Geometry: final body of the model. Coordinates: model frame, mm. Face numbers are marked on the shaded views. Give positions to 0.01 mm unless a question says otherwise; leave off trailing zeros. Loops run counter-clockwise (first coordinate to the right, second up) from the corner with the lowest first, then second, coordinate; pieces in that order, holes last. Notation, with made-up numbers: M -8.5,40.5 L 5.5,40.5 A13 cw 5.5,44.5 Z; hole C -38.75,71 d4. An arc over 180 degrees is marked long. Put each result on its own line as item: value.
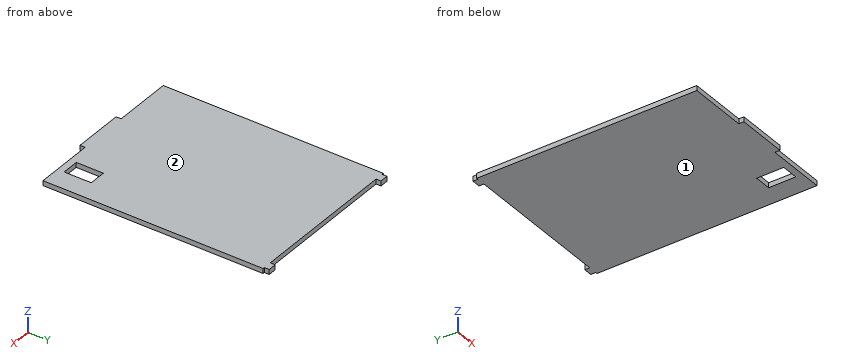
```python
from build123d import *

# Parameters (mm, degrees)
EXTRUDE_1_DEPTH = 2.9


with BuildPart() as part:
    # 草图1 → 凸台-拉伸1 (new body)
    with BuildSketch(Plane.XY):
        Polygon((65, -3), (65, 0), (100, 0), (100, 130), (99, 130), (99, 132.9), (95, 132.9), (94, 132.9), (94, 130), (6, 130), (6, 132.9), (5, 132.9), (1, 132.9), (1, 130), (0, 130), (0, 0), (35, 0), (35, -3), (50, -3), align=None)
        Polygon((83, 4), (78, 4), (78, 20), (83, 20), (88, 20), (88, 4), align=None, mode=Mode.SUBTRACT)
    extrude(amount=EXTRUDE_1_DEPTH)


solid = part.part
```
Item 1: Pin query (flat end, axial travel): pin 1 Ø0.9 at (y, z) = (131.5, 1) entering from -X; pin 2 Ø0.9 at (y, z) = (131.5, 1) entering from +X; pin 3 Ø1.4 at (x, z) = (21, 1) entering from -Y. Return the tip coordinate at first contact, or that it passes through.
Output values:
pin 1: x = 1
pin 2: x = 99
pin 3: y = 0
Item 2: Section C-C on x = 44. Output: boundary loops of the cut face in (y, z).
Output values:
outline: M -3,0 L 130,0 L 130,2.9 L -3,2.9 Z
Item 3: Line query: probe 1 along X at (y, z) = (11.5, 2.25); probe 2 along Y at (x, z) = (84, 1.35); probe 3 along Y at (x, z) = (25.5, 0.65). Output: solid intervals per line, ascending. Write a range as [from, to].
Output values:
probe 1: [0, 78], [88, 100]
probe 2: [0, 4], [20, 130]
probe 3: [0, 130]
Item 4: Section A-A on x = 81. Output: boundary loops of the cut face in (y, z).
Output values:
outline: M 0,0 L 4,0 L 4,2.9 L 0,2.9 Z; M 20,0 L 130,0 L 130,2.9 L 20,2.9 Z
Item 5: Mould query, pull axis Z, two halves, no side actions, for the marked faces 1 and 2. Classes: pulls with the +Z half, pulls with the -Z half, needs draft (parallel to the pull), parting line crosses it, or undercut.
Output values:
face 1: pulls with the -Z half
face 2: pulls with the +Z half
Item 6: Section D-D on x = 30.5. Output: boundary loops of the cut face in (y, z), then the cut area to 3 significant figures.
Output values:
outline: M 0,0 L 130,0 L 130,2.9 L 0,2.9 Z
area: 377 mm²
Item 7: Section B-B on z = 1.7. Output: boundary loops of the cut face in (x, y), then the cut area to 3 significant figures.
Output values:
outline: M 0,0 L 35,0 L 35,-3 L 65,-3 L 65,0 L 100,0 L 100,130 L 99,130 L 99,132.9 L 94,132.9 L 94,130 L 6,130 L 6,132.9 L 1,132.9 L 1,130 L 0,130 Z; hole M 78,4 L 88,4 L 88,20 L 78,20 Z
area: 13,000 mm²
